Part print with two shaded views. Sizes in mm from the minimum x, y, z corner. Coordinates: 2 decimals unless noted, no trailing zeros. Loops run counter-clockwise (first coordinate to the right, second up) from the corner with the lowest first, then second, coordinate; pieces in that order, holes last. Notation, with made-up numbers: (-33, 18) -> (-4, 18) arc R27 ccw to (-4, 47) -> close; hole circle Ø6 at (-22.75, 34.5). An arc over 180 degrees is marked (long way). Return JSON: item names as keys, results as strings. Group by question number.
(1) Saw through at A-A on x = 3.35. Write the cut outline in (y, z).
(2) Flat gauge pins, fed straight in: pin 1 Ø0.8 at (y, z) = (1, 3.5) entering from +X; pin 2 Ø2 at (y, z) = (6.5, 3.5) entering from +X. Where does each tip first touch, or does it go through?
(3) Mould opens along Z. For the marked faces 1, 2 and 3 say: pulls with the +Z half, pulls with the -Z half, needs draft (parallel to the pull), parting line crosses it, or undercut.
(4) Saw through at B-B on z = 1. Give the number of separate pieces and of enclosed holes in the cut face, then the cut area to 3 significant figures.
(5) Saw through at C-C on y = 2. Write the cut outline in (x, z) (1 decimal), then the cut area to 3 significant figures.
(6) Probe L1, parallel to Y at x = 2.95, z = 4.75; L2, parallel to X at y = 1.5, z = 10.25 (1 decimal); L3, parallel to X at y = 4, z = 3.25 (1 decimal). List the from-to ranges inside material, lowest first.
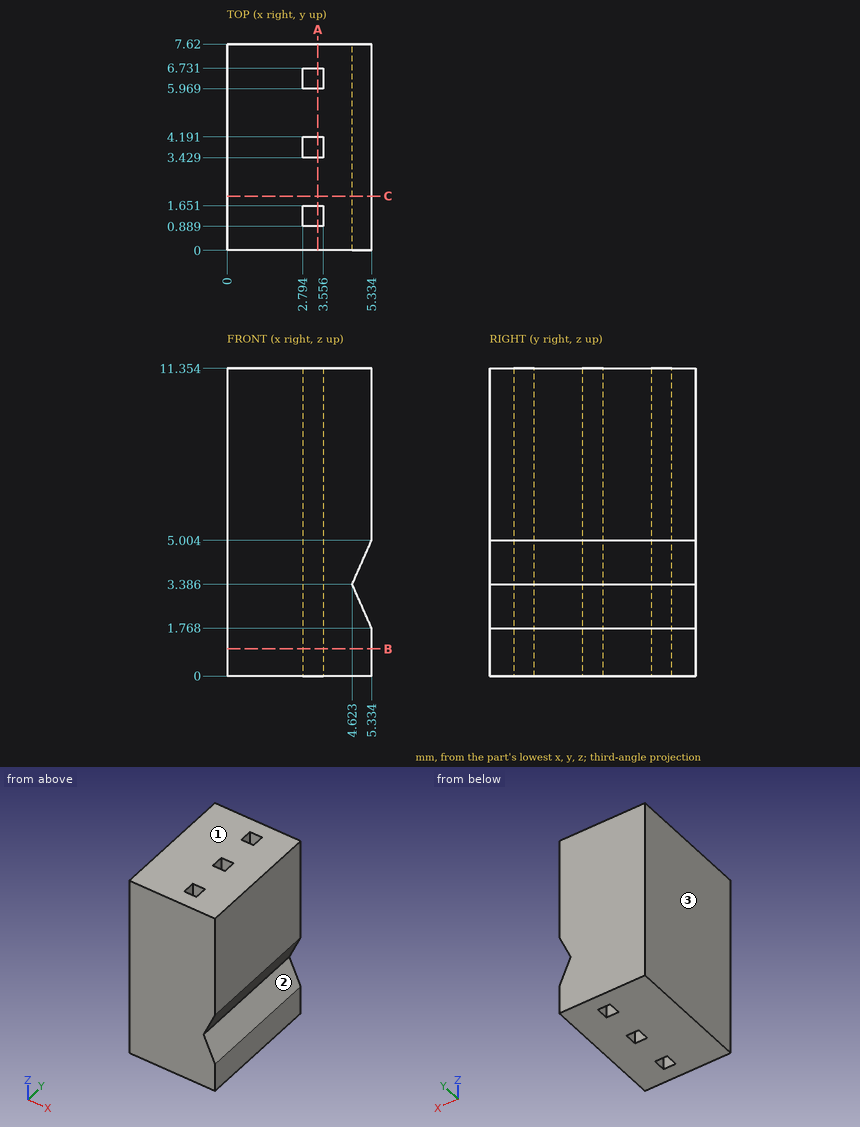
Geometry results:
{
 "1": {"outline": "(0, 0) -> (0.89, 0) -> (0.89, 11.35) -> (0, 11.35) -> close; (1.65, 0) -> (3.43, 0) -> (3.43, 11.35) -> (1.65, 11.35) -> close; (4.19, 0) -> (5.97, 0) -> (5.97, 11.35) -> (4.19, 11.35) -> close; (6.73, 0) -> (7.62, 0) -> (7.62, 11.35) -> (6.73, 11.35) -> close"},
 "2": {"pin 1": "x = 4.85", "pin 2": "x = 5.11"},
 "3": {"face 1": "pulls with the +Z half", "face 2": "undercut", "face 3": "needs draft"},
 "4": {"separate pieces": "1", "enclosed holes": "3", "area": "38.9 mm²"},
 "5": {"outline": "(0, 0) -> (5.3, 0) -> (5.3, 1.8) -> (4.6, 3.4) -> (5.3, 5) -> (5.3, 11.4) -> (0, 11.4) -> close", "area": "59.4 mm²"},
 "6": {"L1": "0 to 0.89, 1.65 to 3.43, 4.19 to 5.97, 6.73 to 7.62", "L2": "0 to 2.8, 3.6 to 5.3", "L3": "0 to 2.8, 3.6 to 4.7"}
}
